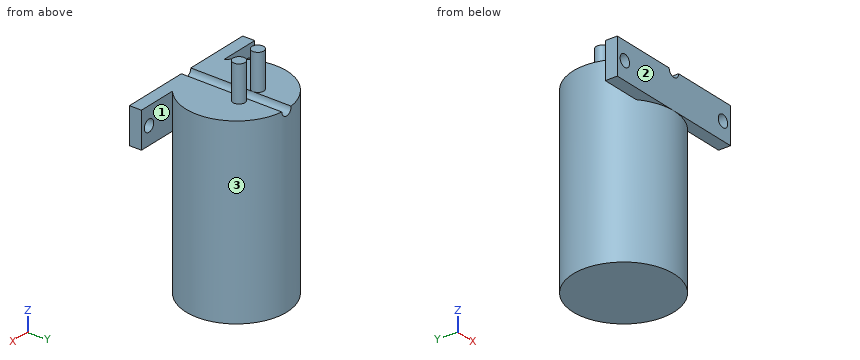
from build123d import *

# Parameters (mm, degrees)
SKETCH1_R                    = 13.335
BOSS_EXTRUDE1_DEPTH          = 48.26
SKETCH2_W                    = 38.1
SKETCH2_H                    = 9.525
BOSS_EXTRUDE2_DEPTH          = 3.175
F_1_8_0_125_DIAMETER_HOLE1_D = 3.175
SKETCH5_R                    = 1.5875
BOSS_EXTRUDE3_DEPTH          = 9.525


with BuildPart() as part:
    # Sketch1 → Boss-Extrude1 (new body)
    with BuildSketch(Plane.XY):
        Circle(SKETCH1_R)
    extrude(amount=BOSS_EXTRUDE1_DEPTH)

    # Sketch2 → Boss-Extrude2 (add)
    with BuildSketch(Plane(origin=(0, -13.335, 0), x_dir=(-1, 0, 0), z_dir=(0, -1, 0))):
        with Locations((0, -43.4975)):
            Rectangle(SKETCH2_W, SKETCH2_H)
    extrude(amount=-BOSS_EXTRUDE2_DEPTH)

    # 1/8 (0.125) Diameter Hole1 (through all)
    with Locations(Plane(origin=(0, -13.335, 0), x_dir=(-1, 0, 0), z_dir=(0, -1, 0))):
        with Locations((-16.51, -43.4975), (16.51, -43.4975), (0, -48.26)):
            Hole(F_1_8_0_125_DIAMETER_HOLE1_D / 2)

    # Sketch5 → Boss-Extrude3 (add)
    with BuildSketch(Plane.XY.offset(48.26)):
        with Locations((-3.175, 3.175)):
            Circle(SKETCH5_R)
        with Locations((3.175, 3.175)):
            Circle(SKETCH5_R)
    extrude(amount=BOSS_EXTRUDE3_DEPTH)


solid = part.part
Work out the finished part from the listing and answer in its coordinate system (mm). Face numbers are marked on the shaded views. A direction names the side the tool comes from. Give positions to 0.01 mm unless a question says otherwise; leave off trailing zeros. Write each loop counter-clockwise with the first axis right and the second up, starting at its lowest first coordinate (ties: lowest second). Pieces come first, ordered by that corner, then holes.
Q1. The part is cut by section B-B on y = 0. Give the vertices of the cut face in (x, z) (1 decimal).
Answer:
outline: (-13.3, 0) - (13.3, 0) - (13.3, 48.3) - (1.6, 48.3) arc R1.6 cw to (-1.6, 48.3) - (-13.3, 48.3) - close
Q2. The part is cut by section A-A on x = 16.51. Give the vertices of the cut face in (y, z) (3 decimals).
Answer:
outline: (-13.335, 38.735) - (-10.16, 38.735) - (-10.16, 41.91) - (-13.335, 41.91) - close; (-13.335, 45.085) - (-10.16, 45.085) - (-10.16, 48.26) - (-13.335, 48.26) - close
Q3. The part is cut by section D-D on x = -16. Give the vertices of the cut face in (y, z) (3 decimals).
Answer:
outline: (-13.335, 38.735) - (-10.16, 38.735) - (-10.16, 41.994) - (-13.335, 41.994) - close; (-13.335, 45.001) - (-10.16, 45.001) - (-10.16, 48.26) - (-13.335, 48.26) - close
Q4. A tool of negligible diameter and unlimited length cuts with its end or side. For the marked faces 1, 2 and 3, from which of +Z, -Z, +X, -X, +Y, -Y can it reach the whole face along a straight path? Write none if from no direction.
Answer:
face 1: +Z, -Z, +X
face 2: +Z, -Z, +X, -X, -Y
face 3: -Z
Q5. Straight lines are drawn through the part: L1, parallel to Z at x = -16.51, y = -11.15 (3 decimals); L2, parallel to Z at x = -3, y = -6.75; L3, parallel to Z at x = -7, y = -11.5 (3 decimals). For each, find the intervals that lie inside material, in ascending order.
Answer:
L1: z = 38.735 to 41.91, 45.085 to 48.26
L2: z = 0 to 48.26
L3: z = 38.735 to 48.26
Q6. The part is cut by section C-C on x = 2.5. Give the vertices of the cut face in (y, z) (3 decimals).
Answer:
outline: (-13.335, 38.735) - (-13.099, 38.735) - (-13.099, 0) - (13.099, 0) - (13.099, 48.26) - (4.612, 48.26) - (4.612, 57.785) - (1.738, 57.785) - (1.738, 48.26) - (-13.335, 48.26) - close
Q7. Given pin 1 (5 mm diameter, centred on x = -10.5, z = 26.5, fed in from -Y); pin 2 (12 mm diameter, centred on x = 13.5, z = 10.5, fed in from -Y); pin 3 (5 mm diameter, centred on x = 12.5, y = -6.5, fed in from +Z); pin 4 (2.5 mm diameter, centred on x = -9.5, y = -11, fed in from -Z), each flat-ended and moving along its own axis, determine where each tip first touches the part or whether it passes through.
Answer:
pin 1: stops at y = -10.67
pin 2: stops at y = -11.03
pin 3: stops at z = 48.26
pin 4: stops at z = 0
